```python
from build123d import *

# Parameters (mm, degrees)
F0_W     = 3
F0_H     = 10
F1_DEPTH = 3


with BuildPart() as f1:
    # F0 (on Front) → F1 (new body)
    with BuildSketch(Plane.XZ):
        Polygon((-16.875, -16.534092), (-46.875, -1.534092), (-46.875, -11.534092), (-46.875, -16.534092), align=None)
        with Locations((-48.375, -6.534092)):
            Rectangle(F0_W, F0_H)
    extrude(amount=F1_DEPTH)


solid = f1.part
```
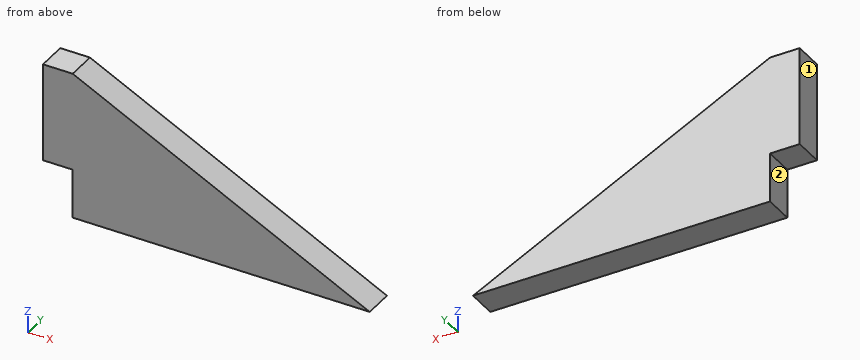
Geometry check sheet. Reference: the model listing, model coordinates, mm. Face numbers are marked on the shaded views. A direction names the side the tool comes from. Coordinates: 2 decimals unless noted, no trailing zeros. Write each loop counter-clockwise with the first axis right and the second up, starting at its lowest first coordinate (ties: lowest second). Pieces come first, ordered by that corner, then holes. Notation, with made-up numbers: M -37.5,-32.5 L -7.5,-32.5 A17 ccw -7.5,-23.5 Z; hole C 30,-1.75 d4. An arc over 180 degrees is marked long. Use one line per item in the form item = value. Start each with the question number.
1) Set-up check for the marked faces 1 and 2: record each of +Z, -Z, +X, -X, +Y, -Y from which the full face is reachable in a straight line by a thin tool's end or side.
2) Section check C-C on z = -7. Enter the section's corners in (x, y) (3 decimals).
3) Section check A-A on y = -0.7. Enter the section's corners in (x, z) (3 decimals).
4) Section check B-B on x = -48. Enter the section's corners in (y, z), and give its area (3 significant figures).
5) Go/stop test with flat-tipped pins: pin 1 Ø1 at (y, z) = (-0.5, -15) entering from -X (3 decimals); pin 2 Ø1 at (y, z) = (-2, -7) entering from +X; pin 3 Ø1 at (x, y) = (-26, -0.5) entering from +Z. Record where each tip stops, or that it passes through.
6) Thickness scan on probe 1 along Z at (x, y) = (-48, -1); probe 2 along Z at (x, y) = (-28.5, -2.75); probe 3 along X at (y, z) = (-1.9, -4.5) (3 decimals). Record the ranges inside material, lowest first. Write a range as from..to.
Responses:
q1.face_1 = +Z, -Z, -X, +Y, -Y
q1.face_2 = -Z, -X, +Y, -Y
q2.outline = M -49.875,-3 L -35.943,-3 L -35.943,0 L -49.875,0 Z
q3.outline = M -49.875,-11.534 L -46.875,-11.534 L -46.875,-16.534 L -16.875,-16.534 L -46.875,-1.534 L -49.875,-1.534 Z
q4.outline = M -3,-11.53 L 0,-11.53 L 0,-1.53 L -3,-1.53 Z
q4.area = 30.0 mm2
q5.pin_1 = -46.875
q5.pin_2 = -34.94
q5.pin_3 = -11.72
q6.probe_1 = -11.53..-1.53
q6.probe_2 = -16.53..-10.72
q6.probe_3 = -49.875..-40.943
